Here's how the part is built. I have some questions about the finished solid (model axes, mm). Face numbers are marked on the shaded views. A direction names the side the tool comes from. Coordinates: 2 decimals unless noted, no trailing zeros. Loops run counter-clockwise (first coordinate to the right, second up) from the corner with the lowest first, then second, coordinate; pieces in that order, holes last. Notation, with made-up numbers: M 58.25,44.25 L 95.25,44.25 A24 ccw 95.25,78.25 Z; hole C 19,-23 d2. An arc over 180 degrees is marked long. Use CSV: the item, a comma, the result in double quotes. Start each with the question number.
Q1. If we section it at A-A (y = 0): Please give me the cut outline in (x, z).
Q2. If we mould it in two halves opening along Y, with no side actions, what happens to the marked faces 1, 2 and 3? For each: +Y half, -Y half, draft (parallel to the pull), parting line (faces both ways), or undercut.
Q3. Please list where these lines run through material, in increasing order: probe 1 along Y at (x, z) = (17.75, -326.5); probe 2 along Y at (x, z) = (0, -321.75); probe 3 along X at (y, z) = (1.5, -326.25). Write a range as [from, to].
Q4. If we section it at B-B (x = 35.5): Please give me the cut outline in (y, z), and give its area (3 significant figures).
Q5. For pin 1 Ø4 at (y, z) = (24.5, -319) entering from -X; pin 2 Ø24 at (x, y) = (0, 0) entering from +Z; pin 3 Ø1 at (x, y) = (-17.5, -11) entering from +Z; pin 4 Ø8.5 at (x, y) = (17.75, 30.74) entering from +Z, each with a flat end and sliding along its axis, tell me the tip position at first contact or that it passes through.
Q6. If we section it at C-C (z = -329.5): State how many separate pieces and enclosed holes the cut face has, and give its area (3 significant figures).
Q7. Which directions (+Z, -Z, +X, -X, +Y, -Y) give clear straight access to the entire face, cutting with the end or side of a thin tool? Please do the marked faces 4 and 5.
from build123d import *

# Parameters (mm, degrees)
STOCK_PPV4_2_START                       = -331
STOCK_PPV4_2_EXTRUDER_MB_1_OUTLINE_R     = 31
STOCK_PPV4_2_EXTRUDER_MB_1_OUTLINE_R_2   = 20
STOCK_PPV4_2_EXTRUDER_MB_1_DEPTH         = 24
STOCK_PPV4_2_EXTRUDER_MB_1_2_OUTLINE_R   = 40
STOCK_PPV4_2_EXTRUDER_MB_1_2_OUTLINE_R_2 = 3.3
STOCK_PPV4_2_EXTRUDER_MB_1_2_OUTLINE_R_3 = 31
STOCK_PPV4_2_EXTRUDER_MB_1_2_DEPTH       = 12
MOVE_FACE1_BY                            = 0.05
MOVE_FACE1_2_BY                          = 0.05
MOVE_FACE1_3_BY                          = 0.05
MOVE_FACE1_4_BY                          = 0.05
MOVE_FACE1_5_BY                          = 0.05
MOVE_FACE1_6_BY                          = 0.05
MOVE_FACE1_7_BY                          = 0.05
MOVE_FACE1_8_BY                          = 0.05
MOVE_FACE1_9_BY                          = 0.05
MOVE_FACE1_10_BY                         = 0.05
MOVE_FACE1_11_BY                         = 0.05
MOVE_FACE1_12_BY                         = 0.05
CHAMFER1_SIZE                            = 3


# Read off the part's stored shape, not the designer's step: Stock-PPV4.2 - Extruder - MB-1
with BuildPart() as part:
    # Stock-PPV4.2 - Extruder - MB-1 outline → Stock-PPV4.2 - Extruder - MB-1 (new body)
    with BuildSketch(Plane.XY.offset(STOCK_PPV4_2_START)):
        Circle(STOCK_PPV4_2_EXTRUDER_MB_1_OUTLINE_R)
        Circle(STOCK_PPV4_2_EXTRUDER_MB_1_OUTLINE_R_2, mode=Mode.SUBTRACT)
    extrude(amount=STOCK_PPV4_2_EXTRUDER_MB_1_DEPTH)

    # Stock-PPV4.2 - Extruder - MB-1 2 outline → Stock-PPV4.2 - Extruder - MB-1 2 (add)
    with BuildSketch(Plane.XY.offset(STOCK_PPV4_2_START)):
        Circle(STOCK_PPV4_2_EXTRUDER_MB_1_2_OUTLINE_R)
        with Locations((-17.75, -30.743901834)):
            Circle(STOCK_PPV4_2_EXTRUDER_MB_1_2_OUTLINE_R_2, mode=Mode.SUBTRACT)
        with Locations((-30.743901834, -17.75)):
            Circle(STOCK_PPV4_2_EXTRUDER_MB_1_2_OUTLINE_R_2, mode=Mode.SUBTRACT)
        with Locations((0, -35.5)):
            Circle(STOCK_PPV4_2_EXTRUDER_MB_1_2_OUTLINE_R_2, mode=Mode.SUBTRACT)
        with Locations((17.75, -30.743901834)):
            Circle(STOCK_PPV4_2_EXTRUDER_MB_1_2_OUTLINE_R_2, mode=Mode.SUBTRACT)
        with Locations((30.743901834, -17.75)):
            Circle(STOCK_PPV4_2_EXTRUDER_MB_1_2_OUTLINE_R_2, mode=Mode.SUBTRACT)
        with Locations((-35.5, 0)):
            Circle(STOCK_PPV4_2_EXTRUDER_MB_1_2_OUTLINE_R_2, mode=Mode.SUBTRACT)
        with Locations((-30.743901834, 17.75)):
            Circle(STOCK_PPV4_2_EXTRUDER_MB_1_2_OUTLINE_R_2, mode=Mode.SUBTRACT)
        with Locations((-17.75, 30.743901834)):
            Circle(STOCK_PPV4_2_EXTRUDER_MB_1_2_OUTLINE_R_2, mode=Mode.SUBTRACT)
        Circle(STOCK_PPV4_2_EXTRUDER_MB_1_2_OUTLINE_R_3, mode=Mode.SUBTRACT)
        with Locations((35.5, 0)):
            Circle(STOCK_PPV4_2_EXTRUDER_MB_1_2_OUTLINE_R_2, mode=Mode.SUBTRACT)
        with Locations((30.743901834, 17.75)):
            Circle(STOCK_PPV4_2_EXTRUDER_MB_1_2_OUTLINE_R_2, mode=Mode.SUBTRACT)
        with Locations((0, 35.5)):
            Circle(STOCK_PPV4_2_EXTRUDER_MB_1_2_OUTLINE_R_2, mode=Mode.SUBTRACT)
        with Locations((17.75, 30.743901834)):
            Circle(STOCK_PPV4_2_EXTRUDER_MB_1_2_OUTLINE_R_2, mode=Mode.SUBTRACT)
    extrude(amount=STOCK_PPV4_2_EXTRUDER_MB_1_2_DEPTH)

    # Move Face1: a curved face moved outward by 0.05
    add(Solid.thicken(part.faces().sort_by_distance((27.443901834, -17.75, -325))[0], MOVE_FACE1_BY))

    # Move Face1 2: a curved face moved outward by 0.05
    add(Solid.thicken(part.faces().sort_by_distance((14.45, -30.743901834, -325))[0], MOVE_FACE1_2_BY))

    # Move Face1 3: a curved face moved outward by 0.05
    add(Solid.thicken(part.faces().sort_by_distance((32.2, 0, -325))[0], MOVE_FACE1_3_BY))

    # Move Face1 4: a curved face moved outward by 0.05
    add(Solid.thicken(part.faces().sort_by_distance((27.443901834, 17.75, -325))[0], MOVE_FACE1_4_BY))

    # Move Face1 5: a curved face moved outward by 0.05
    add(Solid.thicken(part.faces().sort_by_distance((14.45, 30.743901834, -325))[0], MOVE_FACE1_5_BY))

    # Move Face1 6: a curved face moved outward by 0.05
    add(Solid.thicken(part.faces().sort_by_distance((-3.3, 35.5, -325))[0], MOVE_FACE1_6_BY))

    # Move Face1 7: a curved face moved outward by 0.05
    add(Solid.thicken(part.faces().sort_by_distance((-21.05, 30.743901834, -325))[0], MOVE_FACE1_7_BY))

    # Move Face1 8: a curved face moved outward by 0.05
    add(Solid.thicken(part.faces().sort_by_distance((-34.043901834, 17.75, -325))[0], MOVE_FACE1_8_BY))

    # Move Face1 9: a curved face moved outward by 0.05
    add(Solid.thicken(part.faces().sort_by_distance((-38.8, 0, -325))[0], MOVE_FACE1_9_BY))

    # Move Face1 10: a curved face moved outward by 0.05
    add(Solid.thicken(part.faces().sort_by_distance((-34.043901834, -17.75, -325))[0], MOVE_FACE1_10_BY))

    # Move Face1 11: a curved face moved outward by 0.05
    add(Solid.thicken(part.faces().sort_by_distance((-21.05, -30.743901834, -325))[0], MOVE_FACE1_11_BY))

    # Move Face1 12: a curved face moved outward by 0.05
    add(Solid.thicken(part.faces().sort_by_distance((-3.3, -35.5, -325))[0], MOVE_FACE1_12_BY))

    # Chamfer1
    chamfer1_edges = [part.edges().sort_by_distance(p)[0] for p in [
        (-20, 0, -307),
    ]]
    chamfer(chamfer1_edges, length=CHAMFER1_SIZE)


solid = part.part
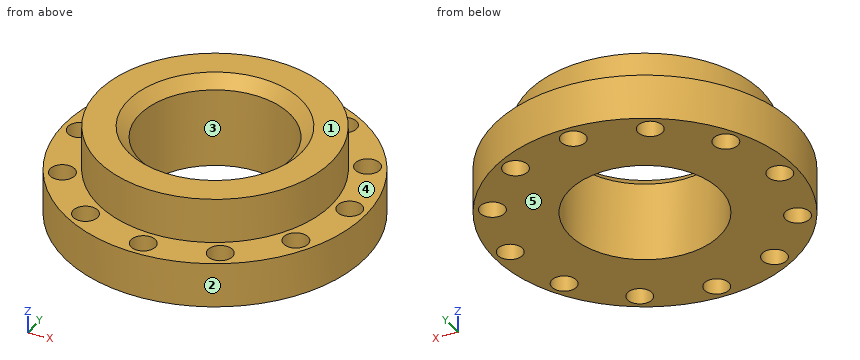
Results below:
1,outline,"M -40,-331 L -38.75,-331 L -38.75,-319 L -40,-319 Z; M -32.25,-331 L -20,-331 L -20,-310 L -23,-307 L -31,-307 L -31,-319 L -32.25,-319 Z; M 20,-331 L 32.25,-331 L 32.25,-319 L 31,-319 L 31,-307 L 23,-307 L 20,-310 Z; M 38.75,-331 L 40,-331 L 40,-319 L 38.75,-319 Z"
2,face 1,"draft"
2,face 2,"parting line"
2,face 3,"undercut"
3,probe 1,"[-35.85, -33.99], [-27.49, -9.22], [9.22, 27.49], [33.99, 35.85]"
3,probe 2,"[-40, -38.75], [-32.25, -20], [20, 32.25], [38.75, 40]"
3,probe 3,"[-39.97, -38.38], [-32.62, -19.94], [19.94, 32.62], [38.38, 39.97]"
4,outline,"M -18.43,-331 L -3.25,-331 L -3.25,-319 L -18.43,-319 Z; M 3.25,-331 L 18.43,-331 L 18.43,-319 L 3.25,-319 Z"
4,area,"364 mm^2"
5,pin 1,"x = -33.07"
5,pin 2,"through"
5,pin 3,"z = -308.83"
5,pin 4,"z = -319"
6,separate pieces,"1"
6,enclosed holes,"13"
6,area,"3,370 mm^2"
7,face 4,"+Z"
7,face 5,"-Z, +X, -X, +Y, -Y"
